Verification items for the finished model (mm, model axes). Face numbers are marked on the shaded views. A direction names the side the tool comes from. Coordinates: 2 decimals unless noted, no trailing zeros. Loops run counter-clockwise (first coordinate to the right, second up) from the corner with the lowest first, then second, coordinate; pieces in that order, holes last. Notation, with made-up numbers: M -26.5,85 L -6.5,85 A25 ccw -6.5,104 Z; hole C -7,5 d2. An arc over 180 degrees is marked long. Write item = value, one per line. Start each with the question number.
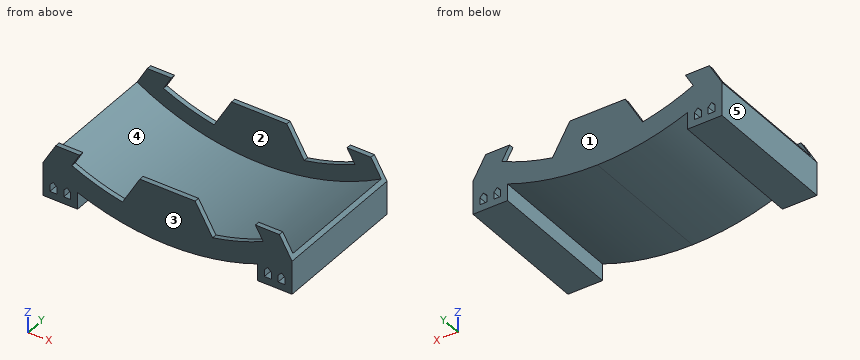
```python
from build123d import *

# Parameters (mm, degrees)
F1_DEPTH  = 127
F2_T      = 4.445
F3_R      = 9.525
F4_DEPTH  = 127
F6_DEPTH  = 127
F8_DEPTH  = 154.94
F10_DEPTH = 4.445
F14_DEPTH = 127


# Not quite as in the source:
# - a shell that OpenCascade refuses in one call is made with other operations: the cavity is built on its own and cut out


with BuildPart() as f1:
    # F0 (on Front) → F1 (new body)
    with BuildSketch(Plane.XZ):
        with BuildLine():
            Line((-19.05, -32.9955678842), (-114.3, -197.9734073051))
            ThreePointArc((-114.3, -197.9734073051), (0, -228.6), (114.3, -197.9734073051))
            Line((114.3, -197.9734073051), (19.05, -32.9955678842))
            ThreePointArc((19.05, -32.9955678842), (32.9955678842, -19.05), (38.1, 0))
            ThreePointArc((38.1, 0), (0, 38.1), (-38.1, 0))
            ThreePointArc((-38.1, 0), (-32.9955678842, -19.05), (-19.05, -32.9955678842))
        make_face()
    extrude(amount=F1_DEPTH)

    # F2: shell of thickness 4.445, made by hand


with BuildPart() as f2_core1:
    # F2_t2: copy of F1
    add(f1.part)

    # the walls: a layer under each face that stays
    f2_faces = [f2_core1.faces().sort_by_distance(p)[0] for p in [
        (0, -127, -95.25),
        (0, 0, -95.25),
        (0, -63.5, -228.6),
        (-32.9955678842, -63.5, -19.05),
    ]]
    thicken(f2_faces, amount=-F2_T, mode=Mode.SUBTRACT)


with BuildPart() as f1_1:
    add(f1.part)

    # what is left inside the walls is the cavity
    f2_cavity = [f2_core1.part.solids().sort_by_distance(p)[0] for p in [
        (0, -122.51055, -136.736667),
    ]]
    add(f2_cavity, mode=Mode.SUBTRACT)

    # F3 (on face) → F4 (cut, through all)
    with BuildSketch(Plane.XZ.offset(127)):
        with BuildLine():
            Line((-50.6196632626, -125.7758286329), (-87.8433632626, -190.2491682786))
            ThreePointArc((-87.8433632626, -190.2491682786), (-48.4057129805, -203.8825383667), (-7.0486462544, -209.4314185741))
            Line((-7.0486462544, -209.4314185741), (-7.0486462544, -169.3468456411))
            Line((-7.0486462544, -169.3468456411), (-50.6196632626, -125.7758286329))
        make_face()
        with BuildLine():
            Line((87.8433632626, -190.2491682786), (50.6196632626, -125.7758286329))
            Line((50.6196632626, -125.7758286329), (7.0486462544, -169.3468456411))
            Line((7.0486462544, -169.3468456411), (7.0486462544, -209.4314185741))
            ThreePointArc((7.0486462544, -209.4314185741), (48.4057129805, -203.8825383667), (87.8433632626, -190.2491682786))
        make_face()
        with BuildLine():
            Line((44.2696632626, -114.7773060049), (7.0486462544, -50.3086134373))
            Line((7.0486462544, -50.3086134373), (7.0486462544, -125.901221947))
            ThreePointArc((7.0486462544, -125.901221947), (11.356209976, -128.3041542134), (14.9024469628, -131.7324762409))
            Line((14.9024469628, -131.7324762409), (44.2696632626, -114.7773060049))
        make_face()
        with BuildLine():
            Line((-7.0486462544, -125.901221947), (-7.0486462544, -50.3086134373))
            Line((-7.0486462544, -50.3086134373), (-44.2696632626, -114.7773060049))
            Line((-44.2696632626, -114.7773060049), (-14.9024469628, -131.7324762409))
            ThreePointArc((-14.9024469628, -131.7324762409), (-11.356209976, -128.3041542134), (-7.0486462544, -125.901221947))
        make_face()
        Circle(F3_R)
    extrude(amount=-F4_DEPTH, mode=Mode.SUBTRACT)

    # F5 (on Front) → F6 (join, through all)
    with BuildSketch(Plane.XZ):
        with BuildLine():
            ThreePointArc((114.3, -197.9734073051), (59.1660337104, -220.8106438897), (0, -228.6))
            Line((0, -228.6), (114.3, -228.6))
            Line((114.3, -228.6), (114.3, -197.9734073051))
        make_face()
        Polygon((95.25, -222.25), (88.9, -222.25), (88.9, -215.9), (92.075, -212.725), (95.25, -215.9), align=None, mode=Mode.SUBTRACT)
        Polygon((107.95, -215.9), (107.95, -222.25), (101.6, -222.25), (101.6, -215.9), (104.775, -212.725), align=None, mode=Mode.SUBTRACT)
        with BuildLine():
            Line((-114.3, -228.6), (0, -228.6))
            ThreePointArc((0, -228.6), (-59.1660337104, -220.8106438897), (-114.3, -197.9734073051))
            Line((-114.3, -197.9734073051), (-114.3, -228.6))
        make_face()
        Polygon((-104.775, -212.725), (-101.6, -215.9), (-101.6, -222.25), (-107.95, -222.25), (-107.95, -215.9), align=None, mode=Mode.SUBTRACT)
        Polygon((-92.075, -212.725), (-88.9, -215.9), (-88.9, -222.25), (-95.25, -222.25), (-95.25, -215.9), align=None, mode=Mode.SUBTRACT)
    extrude(amount=F6_DEPTH)

    # F7 (on Front) → F8 (cut)
    with BuildSketch(Plane.XZ):
        Polygon((-155.1303118467, -177.8), (0, -177.8), (122.5007101893, -177.8), (122.5007101893, 99.952660501), (-155.1303118467, 97.6831391454), align=None)
    extrude(amount=F8_DEPTH, mode=Mode.SUBTRACT)

    # F9 (on face) → F10 (join, through all)
    with BuildSketch(Plane(origin=(0, 0, 0), x_dir=(-1, 0, 0), z_dir=(0, 1, 0))):
        with BuildLine():
            ThreePointArc((-41.3518280797, -205.4293767076), (-65.0419791249, -199.2002596673), (-87.8433632626, -190.2491682786))
            Line((-87.8433632626, -190.2491682786), (-80.6558326058, -177.8))
            Line((-80.6558326058, -177.8), (-102.6528778619, -177.8))
            Line((-102.6528778619, -177.8), (-114.3, -197.9734073051))
            Line((-114.3, -197.9734073051), (-114.3, -228.6))
            Line((-114.3, -228.6), (114.3, -228.6))
            Line((114.3, -228.6), (114.3, -197.9734073051))
            Line((114.3, -197.9734073051), (102.6528778619, -177.8))
            Line((102.6528778619, -177.8), (80.6558326058, -177.8))
            Line((80.6558326058, -177.8), (87.8433632626, -190.2491682786))
            ThreePointArc((87.8433632626, -190.2491682786), (65.0419791249, -199.2002596673), (41.3518280797, -205.4293767076))
            ThreePointArc((41.3518280797, -205.4293767076), (24.2828244592, -208.1382880113), (7.0486462544, -209.4314185741))
            Line((7.0486462544, -209.4314185741), (7.0486462544, -177.8))
            Line((7.0486462544, -177.8), (0, -177.8))
            Line((0, -177.8), (-7.0486462544, -177.8))
            Line((-7.0486462544, -177.8), (-7.0486462544, -209.4314185741))
            ThreePointArc((-7.0486462544, -209.4314185741), (-24.2828244592, -208.1382880113), (-41.3518280797, -205.4293767076))
        make_face()
        Polygon((-107.95, -222.25), (-107.95, -215.9), (-104.775, -212.725), (-101.6, -215.9), (-101.6, -222.25), align=None, mode=Mode.SUBTRACT)
        Polygon((-88.9, -215.9), (-88.9, -222.25), (-95.25, -222.25), (-95.25, -215.9), (-92.075, -212.725), align=None, mode=Mode.SUBTRACT)
        Polygon((88.9, -215.9), (92.075, -212.725), (95.25, -215.9), (95.25, -222.25), (88.9, -222.25), align=None, mode=Mode.SUBTRACT)
        Polygon((101.6, -222.25), (101.6, -215.9), (104.775, -212.725), (107.95, -215.9), (107.95, -222.25), align=None, mode=Mode.SUBTRACT)
        with BuildLine():
            Line((-25.4, -177.8), (-41.3518280797, -205.4293767076))
            ThreePointArc((-41.3518280797, -205.4293767076), (-24.2828244592, -208.1382880113), (-7.0486462544, -209.4314185741))
            Line((-7.0486462544, -209.4314185741), (-7.0486462544, -177.8))
            Line((-7.0486462544, -177.8), (-25.4, -177.8))
        make_face()
        with BuildLine():
            Line((25.4, -177.8), (7.0486462544, -177.8))
            Line((7.0486462544, -177.8), (7.0486462544, -209.4314185741))
            ThreePointArc((7.0486462544, -209.4314185741), (24.2828244592, -208.1382880113), (41.3518280797, -205.4293767076))
            Line((41.3518280797, -205.4293767076), (25.4, -177.8))
        make_face()
    extrude(amount=-F10_DEPTH)

    # F12: F1 across plane


with BuildPart() as f1_2:
    add(f1_1.part)
    add(f1_1.part.mirror(Plane(origin=(0, -63.5, -104.9820841324), x_dir=(1, 0, 0), z_dir=(0, -1, 0))))

    # F13 (on face) → F14 (cut, through all)
    with BuildSketch(Plane.XZ.offset(127)):
        with BuildLine():
            ThreePointArc((0, -228.6), (-41.9894094809, -224.7105905191), (-82.55, -213.1747112113))
            Line((-82.55, -213.1747112113), (-82.55, -228.6))
            Line((-82.55, -228.6), (0, -228.6))
        make_face()
        with BuildLine():
            ThreePointArc((82.55, -213.1747112113), (41.9894094809, -224.7105905191), (0, -228.6))
            Line((0, -228.6), (82.55, -228.6))
            Line((82.55, -228.6), (82.55, -213.1747112113))
        make_face()
    extrude(amount=-F14_DEPTH, mode=Mode.SUBTRACT)


solid = f1_2.part
```
Q1. Sectioned sample at B-B on z = -183.5. Record the cut outline in (x, y) (3 decimals).
Q2. Sectioned sample at D-D on x = -28. Record the cut outline in (y, z) (3 decimals).
Q3. Set-up check for the marked faces 1 and 2: record each of +Z, -Z, +X, -X, +Y, -Y from which the full face is reachable in a straight line by a thin tool's end or side.
Q4. Mould release check, pull along X, two halves, no side actions. Record for the marked faces 3, 4 and 5: +X half, -X half, draft (parallel to the pull), parting line (faces both ways), or undercut.
Q5. Sectioned sample at A-A on y = -51. Count the separate pieces of the cut face and the enclosed holes in it, plus the area to 3 significant figures.
Q6. Gauge pin test, flat ends, axial feed: pin 1 (12 mm diameter, centred on x = 80, y = -65, fed in from +Z); pin 2 (8 mm diameter, centred on x = 85, z = -219.5, fed in from +Y); pin 3 (5 mm diameter, centred on x = -91.5, y = -89.5, fed in from +Z); pin 4 (3 mm diameter, centred on x = -67, y = -79.5, fed in from +Z). Record the tip position at first contact, or that the pin passes through.
Q7. Sectioned sample at C-C on z = -210. Record the cut outline in (x, y) (3 decimals), plus the area to 3 significant figures.
Q8. Scan lines: L1, parallel to Y at x = -6.5, z = -188 (3 decimals); L2, parallel to Z at x = -90, y = -40; L3, parallel to X at y = -112.5, z = -199. Record each from-to range of solid material in increasing order. Write a range as [from, to].
Solutions:
q1.outline = M -105.944,-127 L -83.947,-127 L -83.947,-122.555 L -105.944,-122.555 Z; M -105.944,-4.445 L -83.947,-4.445 L -83.947,0 L -105.944,0 Z; M -28.691,-127 L 28.691,-127 L 28.691,-122.555 L -28.691,-122.555 Z; M -28.691,-4.445 L 28.691,-4.445 L 28.691,0 L -28.691,0 Z; M 83.947,-127 L 105.944,-127 L 105.944,-122.555 L 83.947,-122.555 Z; M 83.947,-4.445 L 105.944,-4.445 L 105.944,0 L 83.947,0 Z
q2.outline = M -127,-226.879 L 0,-226.879 L 0,-182.303 L -4.445,-182.303 L -4.445,-222.399 L -122.555,-222.399 L -122.555,-182.303 L -127,-182.303 Z
q3.face_1 = +Z, -Z, +X, -X, +Y
q3.face_2 = +Z
q4.face_3 = draft
q4.face_4 = undercut
q4.face_5 = -X half
q5.separate_pieces = 1
q5.enclosed_holes = 4
q5.area = 2,280 mm²
q6.pin_1 = -207
q6.pin_2 = 0
q6.pin_3 = -203.49
q6.pin_4 = -213.43
q7.outline = M -114.3,-127 L 114.3,-127 L 114.3,0 L -114.3,0 Z; hole M -78.393,-122.555 L 78.393,-122.555 L 78.393,-4.445 L -78.393,-4.445 Z
q7.area = 10,500 mm²
q8.L1 = [-127, -122.555], [-4.445, 0]
q8.L2 = [-228.6, -222.25], [-214.8, -205.29]
q8.L3 = [-114.3, -103.17], [103.17, 114.3]
